Model file for the job. Use its own axes, mm. Face numbers are marked on the shaded views. A direction names the side the tool comes from. Round coordinates to 2 decimals unless told otherwise and drop trailing zeros. Order: outer loops, then holes, each group sorted by start corner. A loop starts at its lowest first (then second) coordinate and runs counter-clockwise, first axis right, second up. Notation, with made-up numbers: (37, 85.25) -> (68, 85.25) arc R19 cw to (68, 121.25) -> close; hole circle Ø1 at (-25, 40). An arc over 180 degrees is marked (long way). Use CSV: the item, a comma, the result in double quotes.
```python
from build123d import *

# Parameters (mm, degrees)
F1_DEPTH = 9.525
F2_R     = 1.8415
F3_DEPTH = 41.53
F4_DEPTH = 3.175
F5_DEPTH = 5.08
F6_R     = 3.429
F6_R_2   = 1.8415
F7_DEPTH = 2.54
F8_R     = 3.429
F8_R_2   = 1.8415
F9_DEPTH = 2.54


with BuildPart() as f1:
    # F0 (on Top) → F1 (new body)
    with BuildSketch(Plane.XY):
        with BuildLine():
            ThreePointArc((-32.258, 0), (-33.9484276618, 8.5522336929), (-38.7654692948, 15.8182062173))
            ThreePointArc((-38.7654692948, 15.8182062173), (-52.1508813913, 22.3297432037), (-66.6702703397, 19.05))
            ThreePointArc((-66.6702703397, 19.05), (-70.3046684409, 16.2158299298), (-73.2846532478, 12.7))
            Line((-73.2846532478, 12.7), (-64.6795671232, 12.7))
            ThreePointArc((-64.6795671232, 12.7), (-47.6736801053, 14.5001432084), (-38.608, 0))
            ThreePointArc((-38.608, 0), (-47.6736801053, -14.5001432084), (-64.6795671232, -12.7))
            Line((-64.6795671232, -12.7), (-73.2846532478, -12.7))
            ThreePointArc((-73.2846532478, -12.7), (-70.3046684409, -16.2158299298), (-66.6702703397, -19.05))
            ThreePointArc((-66.6702703397, -19.05), (-52.1508813913, -22.3297432037), (-38.7654692948, -15.8182062173))
            ThreePointArc((-38.7654692948, -15.8182062173), (-33.9484276618, -8.5522336929), (-32.258, 0))
        make_face()
        with BuildLine():
            ThreePointArc((-73.2846532478, 12.7), (-70.3046684409, 16.2158299298), (-66.6702703397, 19.05))
            Line((-66.6702703397, 19.05), (-77.216, 19.05))
            Line((-77.216, 19.05), (-77.216, 12.7))
            Line((-77.216, 12.7), (-73.2846532478, 12.7))
        make_face()
        with BuildLine():
            Line((-77.216, -19.05), (-66.6702703397, -19.05))
            ThreePointArc((-66.6702703397, -19.05), (-70.3046684409, -16.2158299298), (-73.2846532478, -12.7))
            Line((-73.2846532478, -12.7), (-77.216, -12.7))
            Line((-77.216, -12.7), (-77.216, -19.05))
        make_face()
        with BuildLine():
            ThreePointArc((-12.7811255343, -14.8039925046), (-19.558, 0), (-12.7811255343, 14.8039925046))
            ThreePointArc((-12.7811255343, 14.8039925046), (-25.9732623614, 10.1879602673), (-38.7654692948, 15.8182062173))
            ThreePointArc((-38.7654692948, 15.8182062173), (-33.9484276618, 8.5522336929), (-32.258, 0))
            ThreePointArc((-32.258, 0), (-33.9484276618, -8.5522336929), (-38.7654692948, -15.8182062173))
            ThreePointArc((-38.7654692948, -15.8182062173), (-25.9732623614, -10.1879602673), (-12.7811255343, -14.8039925046))
        make_face()
        with BuildLine():
            ThreePointArc((8.4395298447, -10.16), (-13.208, 0), (8.4395298447, 10.16))
            Line((8.4395298447, 10.16), (16.711964696, 10.16))
            ThreePointArc((16.711964696, 10.16), (13.9642175742, 13.6936478537), (10.4850018598, 16.51))
            ThreePointArc((10.4850018598, 16.51), (-1.4302661905, 19.5056325871), (-12.7811255343, 14.8039925046))
            ThreePointArc((-12.7811255343, 14.8039925046), (-19.558, 0), (-12.7811255343, -14.8039925046))
            ThreePointArc((-12.7811255343, -14.8039925046), (-1.4302661905, -19.5056325871), (10.4850018598, -16.51))
            ThreePointArc((10.4850018598, -16.51), (13.9642175742, -13.6936478537), (16.711964696, -10.16))
            Line((16.711964696, -10.16), (8.4395298447, -10.16))
        make_face()
        with BuildLine():
            Line((19.558, -10.16), (16.711964696, -10.16))
            ThreePointArc((16.711964696, -10.16), (13.9642175742, -13.6936478537), (10.4850018598, -16.51))
            Line((10.4850018598, -16.51), (19.558, -16.51))
            Line((19.558, -16.51), (19.558, -10.16))
        make_face()
        with BuildLine():
            ThreePointArc((10.4850018598, 16.51), (13.9642175742, 13.6936478537), (16.711964696, 10.16))
            Line((16.711964696, 10.16), (19.558, 10.16))
            Line((19.558, 10.16), (19.558, 16.51))
            Line((19.558, 16.51), (10.4850018598, 16.51))
        make_face()
    extrude(amount=F1_DEPTH)

    # F2 (on face) → F3 (cut, through all)
    with BuildSketch(Plane(origin=(0, 19.05, 0), x_dir=(-1, 0, 0), z_dir=(0, 1, 0))):
        with Locations((71.9431351698, 4.7625)):
            Circle(F2_R)
        with Locations((-15.0215009299, 4.7625)):
            Circle(F2_R)
    extrude(amount=-F3_DEPTH, mode=Mode.SUBTRACT)

    # F2 (on face) → F4 (cut)
    with BuildSketch(Plane(origin=(0, 19.05, 0), x_dir=(-1, 0, 0), z_dir=(0, 1, 0))):
        Polygon((69.67010716, 8.6995), (67.3970791502, 4.7625), (69.67010716, 0.8255), (74.2161631796, 0.8255), (76.4891911894, 4.7625), (74.2161631796, 8.6995), align=None)
        with Locations((71.9431351698, 4.7625)):
            Circle(F2_R, mode=Mode.SUBTRACT)
    extrude(amount=-F4_DEPTH, mode=Mode.SUBTRACT)

    # F2 (on face) → F5 (cut)
    with BuildSketch(Plane(origin=(0, 19.05, 0), x_dir=(-1, 0, 0), z_dir=(0, 1, 0))):
        Polygon((-18.9585009299, 7.0355280098), (-18.9585009299, 2.4894719902), (-15.0215009299, 0.2164439804), (-11.0845009299, 2.4894719902), (-11.0845009299, 7.0355280098), (-15.0215009299, 9.3085560196), align=None)
        with Locations((-15.0215009299, 4.7625)):
            Circle(F2_R, mode=Mode.SUBTRACT)
    extrude(amount=-F5_DEPTH, mode=Mode.SUBTRACT)

    # F6 (on face) → F7 (cut)
    with BuildSketch(Plane.XZ.offset(16.51)):
        with Locations((15.0215009299, 4.7625)):
            Circle(F6_R)
        with Locations((15.0215009299, 4.7625)):
            Circle(F6_R_2, mode=Mode.SUBTRACT)
    extrude(amount=-F7_DEPTH, mode=Mode.SUBTRACT)

    # F8 (on face) → F9 (cut)
    with BuildSketch(Plane.XZ.offset(19.05)):
        with Locations((-71.9431351698, 4.7625)):
            Circle(F8_R)
        with Locations((-71.9431351698, 4.7625)):
            Circle(F8_R_2, mode=Mode.SUBTRACT)
    extrude(amount=-F9_DEPTH, mode=Mode.SUBTRACT)


solid = f1.part
```
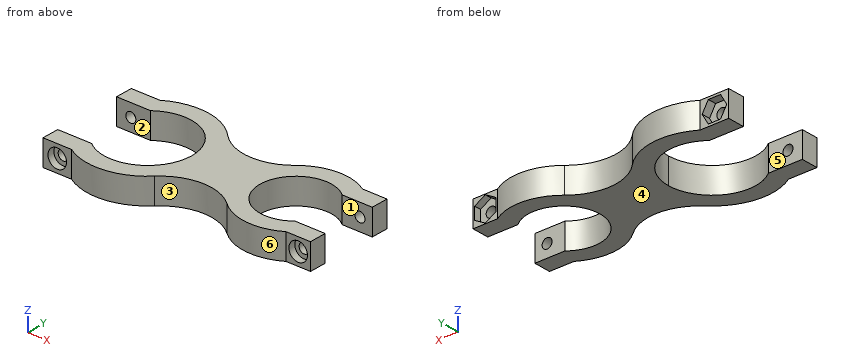
Q1. Cut at A-A (x = 0). Give the cut face in (y, z) (3 decimals).
From the geometry:
outline,"(-19.558, 0) -> (-13.208, 0) -> (-13.208, 9.525) -> (-19.558, 9.525) -> close; (13.208, 0) -> (19.558, 0) -> (19.558, 9.525) -> (13.208, 9.525) -> close"
Q2. Pin check, flat tips, straight feed: pin 1 (3 mm diameter, centred on x = -46.5, z = 1.5, fed in from +Y); pin 2 (2 mm diameter, centred on x = 15.02, z = 4.76, fed in from +Y); pin 3 (5 mm diameter, centred on x = -72, z = 7, fed in from +Y); pin 4 (2.5 mm diameter, centred on x = -70.5, z = 6, fed in from +Y) (3 decimals). Stop position of each tip, or through.
From the geometry:
pin 1,"stops at y = 21.45"
pin 2,"passes through"
pin 3,"stops at y = 19.05"
pin 4,"stops at y = 15.875"
Q3. Cut at C-C (x = -45). Give the cut face in (y, z) (3 decimals).
From the geometry:
outline,"(-20.261, 0) -> (-12.858, 0) -> (-12.858, 9.525) -> (-20.261, 9.525) -> close; (12.858, 0) -> (20.261, 0) -> (20.261, 9.525) -> (12.858, 9.525) -> close"
Q4. Mould opens along Y. For the marked faces 4, 5 and 6 say: +Y half, -Y half, draft (parallel to the pull), parting line (faces both ways), or undercut.
From the geometry:
face 4,"draft"
face 5,"undercut"
face 6,"-Y half"
Q5. Which spindle directions (+Z, -Z, +X, -X, +Y, -Y) get a long thin tool onto all of the face, cutting with end or side? Do the marked faces 1, 2 and 3. Say none if no direction does.
From the geometry:
face 1,"+Z, -Z, +X"
face 2,"+Z, -Z, -X"
face 3,"+Z, -Z, -Y"
Q6. Cut at B-B (x = -71). State how many separate pieces and enclosed holes the cut face has, plus the area to 3 significant figures.
From the geometry:
separate pieces,"4"
enclosed holes,"0"
area,"57.1 mm²"
Q7. Probe line 1 along X through (y, z) = (18, 2); line 2 along X through (y, z) = (14, 7); line 3 along X through (y, z) = (18, 0.75). List the from-to ranges inside material, lowest first.
From the geometry:
line 1,"x = -77.22 to -74.89, -68.99 to -41.27, -7.65 to 7.65"
line 2,"x = -77.22 to -62.75, -46.73 to -36.68, -13.78 to 11.08, 18.96 to 19.56"
line 3,"x = -77.22 to -41.27, -7.65 to 7.65"
Q8. Cut at D-D (y = 1.5). Give the cut face in (x, z) (3 decimals), plus the area to 3 significant figures.
From the geometry:
outline,"(-38.678, 0) -> (-13.123, 0) -> (-13.123, 9.525) -> (-38.678, 9.525) -> close"
area,"243 mm²"
